Part model, mm, in its own coordinate system. A direction names the side the tool comes from. Round coordinates to 2 decimals unless told otherwise and drop trailing zeros. Loops run counter-clockwise (first coordinate to the right, second up) from the corner with the lowest first, then second, coordinate; pieces in that order, holes last. Notation, with made-up numbers: (2.25, 65.5) - (18.25, 65.5) arc R22 ccw to (18.25, 95.5) - close; hole circle Ø8 at (13, -18.5). An arc over 180 degrees is marked (long way). Write each question's results on one line, items separated by ' | '. Start each with the question number.
(1) Flat gauge pins, fed straight in: P1, Ø13, axis at x = 24, z = -14, coming from the +Y side; P2, Ø5, axis at y = 37.5, z = -14.5, coming from the +X side; P3, Ø8, axis at x = 11.5, z = -5.5, coming from the +Y side. Where does each tip first touch, or does it go through?
(2) Cut at C-C, the plane x = 10.75. List the corners of the cut face in (y, z).
(3) Cut at D-D, the plane z = -11.5. List the corners of the cut face in (x, y), then the cut area to 3 significant figures.
(4) Tool access for faces 1 (the face through (29, 2.5, -18)), 2 (the face through (2, 30, -26.054)), 3 (the face through (17, 20, -17)): list every direction of +Z, -Z, +X, -X, +Y, -Y with a clear straight run to the whole face (end or side of a thin tool).
(5) Drill centre lines: L1, parallel to X at y = 1.75, z = -17.5; L2, parallel to Z at x = 3, y = 31; L3, parallel to X at y = 8.5, z = -28.5. Where is each one in solid material? Low to high.
(6) Mould opens along Z. For faces 4 (the face through (35, 1, -17)), 5 (the face through (2, 12.5, -18)), 6 (the face through (4, 22, 0)), 7 (the face through (19.25, 1, -17)) say: released by +Z, released by -Z, zero draft, split by the parting line, or undercut.
(7) Cut at B-B, the plane z = -17.5. List the corners of the cut face in (x, y), then the cut area to 3 significant figures.
(8) Cut at A-A, the plane y = 30. List the corners of the cut face in (x, z).
from build123d import *

# Parameters (mm, degrees)
SKETCH1_W           = 35
SKETCH1_H           = 35
BOSS_EXTRUDE1_DEPTH = 2.5
SKETCH2_W           = 5
SKETCH2_H           = 35
BOSS_EXTRUDE2_DEPTH = 50
SKETCH5_W           = 17
SKETCH5_H           = 35
CUT_EXTRUDE2_DEPTH  = 4
SKETCH6_R           = 5
CUT_EXTRUDE3_DEPTH  = 10
SKETCH7_W           = 2
SKETCH7_H           = 35
BOSS_EXTRUDE3_DEPTH = 35
SKETCH8_W           = 7.3
SKETCH8_H           = 15.5
CUT_EXTRUDE4_DEPTH  = 3.5


with BuildPart() as part:
    # Sketch1 → Boss-Extrude1 (new body)
    with BuildSketch(Plane(origin=(0, 0, 0), x_dir=(1, 0, 0), z_dir=(0, 1, 0))):
        with Locations((17.5, 17.5)):
            Rectangle(SKETCH1_W, SKETCH1_H)
    extrude(amount=BOSS_EXTRUDE1_DEPTH)

    # Sketch2 → Boss-Extrude2 (add)
    with BuildSketch(Plane(origin=(0, 2.5, 0), x_dir=(1, 0, 0), z_dir=(0, 1, 0))):
        with Locations((2.5, 17.5)):
            Rectangle(SKETCH2_W, SKETCH2_H)
    extrude(amount=BOSS_EXTRUDE2_DEPTH)

    # Sketch5 → Cut-Extrude2 (cut)
    with BuildSketch(Plane.ZY):
        with Locations((-17.553851225, 30)):
            Rectangle(SKETCH5_W, SKETCH5_H)
    extrude(amount=-CUT_EXTRUDE2_DEPTH, mode=Mode.SUBTRACT)

    # Sketch6 → Cut-Extrude3 (cut)
    with BuildSketch(Plane(origin=(0, 2.5, 0), x_dir=(1, 0, 0), z_dir=(0, 1, 0))):
        with Locations((10.75, 17.5)):
            Circle(SKETCH6_R)
    extrude(amount=-CUT_EXTRUDE3_DEPTH, mode=Mode.SUBTRACT)

    # Sketch7 → Boss-Extrude3 (add)
    with BuildSketch(Plane(origin=(0, 2.5, 0), x_dir=(1, 0, 0), z_dir=(0, 1, 0))):
        with Locations((18, 17.5)):
            Rectangle(SKETCH7_W, SKETCH7_H)
    extrude(amount=BOSS_EXTRUDE3_DEPTH)

    # Sketch8 → Cut-Extrude4 (cut, through all)
    with BuildSketch(Plane(origin=(0, 2.5, 0), x_dir=(1, 0, 0), z_dir=(0, 1, 0))):
        with Locations((22.9, 17.5)):
            Rectangle(SKETCH8_W, SKETCH8_H)
    extrude(amount=-CUT_EXTRUDE4_DEPTH, mode=Mode.SUBTRACT)


solid = part.part
A:
1) P1: y = 37.5 | P2: x = 19 | P3: y = 2.5
2) outline: (0, -35) - (2.5, -35) - (2.5, -22.5) - (0, -22.5) - close; (0, -12.5) - (2.5, -12.5) - (2.5, 0) - (0, 0) - close
3) outline: (0, 0) - (19.25, 0) - (19.25, 2.5) - (19, 2.5) - (19, 37.5) - (17, 37.5) - (17, 2.5) - (5, 2.5) - (5, 52.5) - (0, 52.5) - (0, 47.5) - (4, 47.5) - (4, 12.5) - (0, 12.5) - close; (26.55, 0) - (35, 0) - (35, 2.5) - (26.55, 2.5) - close | area: 249 mm2
4) face 1: +Z, -Z, +X, +Y | face 2: -X | face 3: +Z, -Z, +Y
5) L1: 0 to 5.75, 15.75 to 19.25, 26.55 to 35 | L2: -35 to -26.05, -9.05 to 0 | L3: 0 to 5, 17 to 19
6) face 4: zero draft | face 5: undercut | face 6: released by +Z | face 7: undercut
7) outline: (0, 0) - (5.75, 0) - (5.75, 2.5) - (5, 2.5) - (5, 52.5) - (0, 52.5) - (0, 47.5) - (4, 47.5) - (4, 12.5) - (0, 12.5) - close; (15.75, 0) - (19.25, 0) - (19.25, 2.5) - (19, 2.5) - (19, 37.5) - (17, 37.5) - (17, 2.5) - (15.75, 2.5) - close; (26.55, 0) - (35, 0) - (35, 2.5) - (26.55, 2.5) - close | area: 224 mm2
8) outline: (0, -35) - (5, -35) - (5, 0) - (0, 0) - (0, -9.05) - (4, -9.05) - (4, -26.05) - (0, -26.05) - close; (17, -35) - (19, -35) - (19, 0) - (17, 0) - close
